```python
from build123d import *

# Parameters (mm, degrees)
F3_DEPTH = 2
F5_DEPTH = 2
F6_W     = 85
F6_H     = 100
F6_R     = 4.5
F6_R_2   = 12.5
F7_DEPTH = 2


with BuildPart() as f1:
    # F0 (on Front) → F1 (revolve)
    with BuildSketch(Plane.XZ):
        Polygon((16, 5), (10, 5), (10, 35), (15, 35), (15, 50), (-15, 50), (-15, 35), (-10, 35), (-10, 5), (-16, 5), (-16, 0), (16, 0), align=None)
    revolve(axis=Axis((0, 0, 0), (1, 0, 0)))

    # F2 (on face) → F3 (join)
    with BuildSketch(Plane(origin=(-16, 0, 0), x_dir=(0, -1, 0), z_dir=(-1, 0, 0))):
        with BuildLine():
            Line((6, 73), (-7.5, 0))
            ThreePointArc((-7.5, 0), (-2.426055, -7.096778), (5.930469, -4.591246))
            Line((5.930469, -4.591246), (66, 73))
            Line((66, 73), (6, 73))
        make_face()
    extrude(amount=F3_DEPTH)

    # F4 (on face) → F5 (join)
    with BuildSketch(Plane.YZ.offset(16)):
        with BuildLine():
            ThreePointArc((-5.930469, -4.591246), (2.426055, -7.096778), (7.5, 0))
            Line((7.5, 0), (-6, 73))
            Line((-6, 73), (-66, 73))
            Line((-66, 73), (-5.930469, -4.591246))
        make_face()
    extrude(amount=F5_DEPTH)

    # F6 (on face) → F7 (join)
    with BuildSketch(Plane.XY.offset(73)):
        with Locations((0, -36)):
            Rectangle(F6_W, F6_H)
        with Locations((-30, -76)):
            Circle(F6_R, mode=Mode.SUBTRACT)
        with Locations((30, -76)):
            Circle(F6_R, mode=Mode.SUBTRACT)
        with Locations((-30, 4)):
            Circle(F6_R, mode=Mode.SUBTRACT)
        with Locations((0, -36)):
            Circle(F6_R_2, mode=Mode.SUBTRACT)
        with Locations((30, 4)):
            Circle(F6_R, mode=Mode.SUBTRACT)
    extrude(amount=F7_DEPTH)


solid = f1.part
```
Geometry: final body of the model. Coordinates: model frame, mm. A direction names the side the tool comes from. Round coordinates to 2 decimals unless told otherwise and drop trailing zeros. Order: outer loops, then holes, each group sorted by start corner. A loop starts at its lowest first (then second) coordinate and runs counter-clockwise, first axis right, second up. Notation, with made-up numbers: M 60.5,-7.5 L 105.5,-7.5 A33 cw 105.5,22.5 Z; hole C 65,-26 d11. An arc over 180 degrees is marked long. One line per item, written item: value.
(1) Cut plane D-D (y = -16). Return the cut outline in (x, z).
Result sheet:
outline: M -42.5,73 L -18,73 L -18,8.42 L -16,8.42 L -16,73 L 16,73 L 16,8.42 L 18,8.42 L 18,73 L 42.5,73 L 42.5,75 L -42.5,75 Z; M -15,-47.37 L 15,-47.37 L 15,-31.13 L 10,-31.13 L 10,31.13 L 15,31.13 L 15,47.37 L -15,47.37 L -15,31.13 L -10,31.13 L -10,-31.13 L -15,-31.13 Z
(2) Cut plane B-B (y = -76). Return the cut outline in (x, z), and give its area (3 significant figures).
Result sheet:
outline: M -42.5,73 L -34.5,73 L -34.5,75 L -42.5,75 Z; M -25.5,73 L 25.5,73 L 25.5,75 L -25.5,75 Z; M 34.5,73 L 42.5,73 L 42.5,75 L 34.5,75 Z
area: 134 mm2
(3) Reachability of faces 1 (the flat face through (-18, -21, 42)), 2 (the flat face through (-16.986, 0.656, 37.011)), 3 (the cylindrical face through (16.99, 2.3, -7.14)) from +Z, -Z, +X, -X, +Y, -Y: full face, straight path, thin tool, end or side. Return the list, or none.
Result sheet:
face 1: -Z, -X, +Y, -Y
face 2: -X, +Y
face 3: -Z, +X
(4) Pin query (flat end, axial travel): P1, Ø1.5, axis at y = -22.5, z = 1.5, coming from the -X side; P2, Ø1.5, axis at y = 33, z = 15, coming from the -X side; P3, Ø5, axis at x = 12.5, z = 19.5, coming from the +Y side. Return the tip coordinate at first contact, or that it passes through.
Result sheet:
P1: x = -10
P2: x = -15
P3: y = 47.02
(5) Pull-direction query (Y, two-part tool) for faces 4 (the cylindrical face through (-25.84, 2.28, 73.99)), 5 (the cylindrical face through (-16.986, 2.549, -7.054)), 6 (the flat face through (15, 10, 34)); classes: pulls with the +Y half, pulls with the -Y half, needs draft (parallel to the pull), parting line crosses it, or undercut.
Result sheet:
face 4: undercut
face 5: parting line crosses it
face 6: needs draft
(6) Cut plane A-A (x = 30). Return the cut outline in (y, z).
Result sheet:
outline: M -86,73 L -80.5,73 L -80.5,75 L -86,75 Z; M -71.5,73 L -0.5,73 L -0.5,75 L -71.5,75 Z; M 8.5,73 L 14,73 L 14,75 L 8.5,75 Z
(7) Line query: probe 1 along Y at (x, z) = (12.7, 0); probe 2 along Y at (x, z) = (-30, 73.5); probe 3 along X at (y, z) = (-1, 40.5). Output: solid intervals per line, ascending. Write a range as [from, to].
Result sheet:
probe 1: [-50, -35], [-5, 5], [35, 50]
probe 2: [-86, -80.5], [-71.5, -0.5], [8.5, 14]
probe 3: [-18, -16], [-15, 15], [16, 18]
(8) Cut plane C-C (z = 8.5). Return the cut outline in (x, y).
Result sheet:
outline: M -18,-16.07 L -16,-16.07 L -16,5.93 L -18,5.93 Z; M -15,-49.27 L 15,-49.27 L 15,-33.95 L 10,-33.95 L 10,33.95 L 15,33.95 L 15,49.27 L -15,49.27 L -15,33.95 L -10,33.95 L -10,-33.95 L -15,-33.95 Z; M 16,-16.07 L 18,-16.07 L 18,5.93 L 16,5.93 Z
